from build123d import *

# Parameters (mm, degrees)
F0_W          = 25.4
F0_H          = 25.4
F1_DEPTH      = 3.175
F1_TAPER      = -3
F3_W          = 5.08
F3_H          = 12.7
F6_DEPTH      = 6.35
F6_DEPTH_BACK = 6.35
F7_R          = 5.08
F8_R          = 1.524


with BuildPart() as f1:
    # F0 (on Top) → F1 (new body)
    with BuildSketch(Plane.XY):
        Rectangle(F0_W, F0_H)
    extrude(amount=F1_DEPTH, taper=F1_TAPER)

    # F4: sweep along a path in F2
    with BuildLine(Plane.XZ) as f4_path:
        ThreePointArc((-10.16, 0), (0, -23.5582897328), (10.16, 0))
    # F3 (on face) → F4 (sweep)
    with BuildSketch(Plane(origin=(0, 0, 0), x_dir=(1, 0, 0), z_dir=(0, 0, -1))):
        with Locations((-10.16, 0)):
            Rectangle(F3_W, F3_H)
    sweep(path=f4_path.line)

    # F5 (on Front) → F6 (join, two sides)
    with BuildSketch(Plane.XZ) as f6_sk:
        with BuildLine():
            Line((10.0130578512, -2.535746045), (10.16, 0))
            Line((10.16, 0), (7.62, 0))
            ThreePointArc((7.62, 0), (8.9072265211, -1.1822790439), (10.0130578512, -2.535746045))
        make_face()
    extrude(amount=F6_DEPTH)
    extrude(f6_sk.sketch, amount=-F6_DEPTH_BACK)

    # F7
    f7_edges = [f1.edges().sort_by_distance(p)[0] for p in [
        (-12.783197, -12.783197, 1.5875),
        (-12.783197, 12.783197, 1.5875),
        (12.783197, 12.783197, 1.5875),
        (12.783197, -12.783197, 1.5875),
    ]]
    fillet(f7_edges, radius=F7_R)

    # F8
    f8_edges = [f1.edges().sort_by_distance(p)[0] for p in [
        (-1.743325, -6.35, -21.711017),
        (8.907227, -6.35, -1.182279),
        (-1.743325, 6.35, -21.711017),
        (0, 6.35, -25.501344),
        (0, -6.35, -25.501344),
        (8.907227, 6.35, -1.182279),
    ]]
    fillet(f8_edges, radius=F8_R)


solid = f1.part
Part model, mm, in its own coordinate system. A direction names the side the tool comes from. Coordinates: 2 decimals unless noted, no trailing zeros. Put each result on its own line as item: value.
1. Flat gauge pins, fed straight in: pin 1 Ø1.5 at (x, z) = (12, -15.5) entering from -Y; pin 2 Ø7.5 at (x, y) = (2.5, 3.5) entering from -Z; pin 3 Ø12 at (y, z) = (1, -21.5) entering from +X; pin 4 Ø2 at (x, y) = (-6, 0) entering from -Z. Where does each tip first touch, or does it go through?
Final values:
pin 1: stops at y = -6.35
pin 2: stops at z = -25.5
pin 3: stops at x = 14.77
pin 4: stops at z = -24.7
2. 3-axis set-ups, long thin cutter, end or side, ignore diameter. For faces 1 (the flat face through (1, 6.35, -23.5)), 2 (the flat face through (0, 0, 3.175)): which of +Z, -Z, +X, -X, +Y, -Y reach the whole face in a straight line?
Final values:
face 1: -Z, +X, -X, +Y
face 2: +Z, +X, -X, +Y, -Y
3. Probe line 1 along Z through (x, y) = (0, 0.25) (3 decimals); line 2 along Z through (x, y) = (-10.5, -10) (3 decimals); line 3 along Z through (x, y) = (-3, -1.25) (3 decimals). List the from-to ranges inside material, lowest first. Write a range as [from, to].
Final values:
line 1: z = [-25.501, -21.836], [0, 3.175]
line 2: z = [0, 3.175]
line 3: z = [-25.216, -21.463], [0, 3.175]
4. Two-plate mould, pull along X, no slides. Class faces 3 (the flat face through (0, 0, 0)), 4 (the cylindrical face through (-0.494, 0.068, -25.494)), 5 (the flat face through (1, -6.35, -23.5)): +X half, -X half, draft (parallel to the pull), parting line (faces both ways), or undercut.
Final values:
face 3: undercut
face 4: parting line
face 5: draft
